Build history of the part. All positions in model axes, mm. A direction names the side the tool comes from. Give positions to 0.01 mm unless a question says otherwise; leave off trailing zeros. Write each loop counter-clockwise with the first axis right and the second up, starting at its lowest first coordinate (ties: lowest second). Pieces come first, ordered by that corner, then holes. Notation, with made-up numbers: M -4.5,67 L 17.5,67 A14 ccw 17.5,71 Z; hole C 63.5,-15.5 d6. An arc over 180 degrees is marked long. One line per item, written item: value. Start each with the question number.
Autodesk Inventor part; units mm, degrees
ref_plane "YZ Plane" through (0, 0, 0) normal (1, 0, 0) x (0, 1, 0)
ref_plane "XZ Plane" through (0, 0, 0) normal (0, 1, 0) x (-1, 0, 0)
ref_plane "XY Plane" through (0, 0, 0) normal (0, 0, 1) x (1, 0, 0)
sketch "スケッチ1" plane through (0, 0, 0) normal (0, 0, 1) x (1, 0, 0)
  line L0 (0, 0) -> (27, 0) construction
  line L1 (27, 0) -> (27, 5) construction
  line L2 (27, 5) -> (0, 5) construction
  line L3 (0, 5) -> (0, 0) construction
  line L4 (0, 2.5) -> (27, 2.5) construction
  line L5 (13.5, 5) -> (13.5, 0) construction
  circle A0 centre (3.7, 2.5) radius 1.55
  line L6 (7.5, 5) -> (7.5, 0) construction
  circle A1 centre (23.3, 2.5) radius 1.55
  line L7 (19.5, 5) -> (19.5, 0) construction
  line L8 (7.49, 5.01) -> (9.59, 5.01) construction
  line L9 (19.51, 5.01) -> (19.51, 2.49)
  line L10 (19.51, 2.49) -> (7.49, 2.49)
  line L11 (7.49, 2.49) -> (7.49, 5.01)
  line L12 (7.49, 5.01) -> (19.51, 2.49) construction
  line L13 (19.51, 5.01) -> (7.49, 2.49) construction
  arc A2 (9.59, 5.01) -> (7.49, 5.01) centre (8.54, 5.01) ccw
  arc A3 (19.51, 5.01) -> (17.41, 5.01) centre (18.46, 5.01) ccw
  line L14 (9.59, 5.01) -> (17.41, 5.01)
  line L15 (9.59, 2.49) -> (7.49, 2.49)
  line L16 (17.41, 5.01) -> (19.51, 5.01) construction
  line L17 (27, 7) -> (0, 7) construction
  line L18 (0, 0) -> (0, 7)
  line L19 (12.1912, 35) -> (37.1912, 35) construction
  line L20 (37.1912, 35) -> (37.1912, 40) construction
  line L21 (37.1912, 40) -> (12.1912, 40) construction
  line L22 (12.1912, 40) -> (12.1912, 35) construction
  line L23 (12.1912, 37.5) -> (37.1912, 37.5) construction
  line L24 (24.6912, 40) -> (24.6912, 35) construction
  circle A4 centre (14.8912, 37.5) radius 1.55
  line L25 (18.6912, 40) -> (18.6912, 35) construction
  line L26 (30.6912, 40) -> (30.6912, 35) construction
  circle A5 centre (34.4912, 37.5) radius 1.55
  line L27 (18.6812, 40.01) -> (20.7812, 40.01) construction
  line L28 (30.7012, 40.01) -> (30.7012, 34.99)
  line L29 (30.7012, 34.99) -> (28.6012, 34.99) construction
  line L30 (18.6812, 34.99) -> (18.6812, 40.01)
  line L31 (18.6812, 40.01) -> (30.7012, 34.99) construction
  line L32 (30.7012, 40.01) -> (18.6812, 34.99) construction
  arc A6 (20.7812, 40.01) -> (18.6812, 40.01) centre (19.7312, 40.01) ccw
  arc A7 (18.6812, 34.99) -> (20.7812, 34.99) centre (19.7312, 34.99) ccw
  arc A8 (30.7012, 40.01) -> (28.6012, 40.01) centre (29.6512, 40.01) ccw
  arc A9 (28.6012, 34.99) -> (30.7012, 34.99) centre (29.6512, 34.99) ccw
  line L33 (20.7812, 40.01) -> (28.6012, 40.01)
  line L34 (20.7812, 34.99) -> (18.6812, 34.99) construction
  line L35 (28.6012, 40.01) -> (30.7012, 40.01) construction
  line L36 (28.6012, 34.99) -> (20.7812, 34.99)
  line L37 (12.1912, 73) -> (12.1912, 68) construction
  circle A10 centre (14.8912, 70.5) radius 1.55
  line L38 (37.1912, 68) -> (37.1912, 73) construction
  line L39 (30.6912, 73) -> (30.6912, 68) construction
  circle A11 centre (34.4912, 70.5) radius 1.55
  line L40 (30.7012, 73.01) -> (30.7012, 67.99)
  line L41 (18.6912, 73) -> (18.6912, 68) construction
  line L42 (12.1912, 68) -> (37.1912, 68) construction
  line L43 (37.1912, 73) -> (12.1912, 73) construction
  line L44 (12.1912, 70.5) -> (37.1912, 70.5) construction
  line L45 (24.6912, 73) -> (24.6912, 68) construction
  line L46 (20.7812, 73.01) -> (28.6012, 73.01)
  line L47 (28.6012, 67.99) -> (20.7812, 67.99)
  line L48 (18.6812, 73.01) -> (30.7012, 67.99) construction
  line L49 (30.7012, 73.01) -> (18.6812, 67.99) construction
  arc A12 (30.7012, 73.01) -> (28.6012, 73.01) centre (29.6512, 73.01) ccw
  line L50 (28.6012, 73.01) -> (30.7012, 73.01) construction
  arc A13 (28.6012, 67.99) -> (30.7012, 67.99) centre (29.6512, 67.99) ccw
  line L51 (30.7012, 67.99) -> (28.6012, 67.99) construction
  line L52 (18.6812, 73.01) -> (20.7812, 73.01) construction
  line L53 (20.7812, 67.99) -> (18.6812, 67.99) construction
  arc A14 (20.7812, 73.01) -> (18.6812, 73.01) centre (19.7312, 73.01) ccw
  arc A15 (18.6812, 67.99) -> (20.7812, 67.99) centre (19.7312, 67.99) ccw
  line L54 (18.6812, 67.99) -> (18.6812, 73.01)
  line L55 (27, 0) -> (27, 6.6473)
  line L56 (37.1912, 35) -> (27.1206, 7.3314)
  line L57 (11.8992, 39.6929) -> (0, 7)
  line L58 (37.1912, 35) -> (37.1912, 73)
  line L59 (6.8054, 101.4338) -> (6.7491, 101.3865)
  arc A16 (4.7394, 86.3065) -> (5.3203, 95.7003) centre (-4.8938, 91.617) ccw
  circle A17 centre (-4.8938, 91.617) radius 14.6063 construction
  line L60 (1.0459, 61.9185) -> (-21.5815, 84.5459) construction
  line L61 (-21.5815, 84.5459) -> (-18.0459, 88.0815) construction
  line L62 (-18.0459, 88.0815) -> (4.5815, 65.4541) construction
  line L63 (4.5815, 65.4541) -> (1.0459, 61.9185) construction
  line L64 (1.0459, 61.9185) -> (-18.0459, 88.0815) construction
  line L65 (-21.5815, 84.5459) -> (4.5815, 65.4541) construction
  line L66 (13.8495, 100.8175) -> (37.1912, 73)
  arc A18 (11.8992, 39.6929) -> (5.2055, 80.7796) centre (-28.1256, 54.2607) ccw
  arc A19 (8.344, 97.7899) -> (6.2953, 101.0057) centre (-4.8938, 91.617) ccw construction
  arc A20 (5.0756, 80.942) -> (7.4988, 83.886) centre (-4.8938, 91.617) ccw construction
  circle A21 centre (8.344, 97.7899) radius 1.55
  circle A22 centre (7.4988, 83.886) radius 1.65
  arc A23 (13.8495, 100.8175) -> (6.8054, 101.4338) centre (10.0193, 97.6035) ccw
  arc A24 (6.7491, 101.3865) -> (5.3203, 95.7003) centre (9.9631, 97.5563) ccw
  arc A25 (4.7394, 86.3065) -> (5.2055, 80.7796) centre (9.1182, 83.8926) ccw
  arc A26 (27.1206, 7.3314) -> (27, 6.6473) centre (29, 6.6473) ccw
  arc A27 (7.49, 3.9749) -> (8.9749, 2.49) centre (8.2325, 3.2325) ccw
  arc A28 (18.0251, 2.49) -> (19.51, 3.9749) centre (18.7675, 3.2325) ccw
  line L67 (0, 0) -> (7.5, -0.5)
  line L68 (7.5, -0.5) -> (19.5, -0.5)
  line L69 (27, 0) -> (19.5, -0.5)
  point P0 (24.6912, 37.5)
  point P1 (24.6912, 70.5)
  point P2 (10.6356, 104.6477)
  point P3 (3.5327, 98.6877)
  point P4 (-8.5, 75)
  point P5 (19.51, 3.9749)
  point P6 (18.0251, 2.49)
  point P7 (5.8711, 81.4297)
  dimension "d0" = 27
  dimension "d1" = 5
  dimension "d2" = 3.1
  dimension "d3" = 12
  dimension "d4" = 19.6
  dimension "d9" = 1.05
  dimension "d10" = 7
  dimension "d11" = 25
  dimension "d12" = 5
  dimension "d13" = 3.1
  dimension "d14" = 12
  dimension "d15" = 19.6
  dimension "d16" = 0.01
  dimension "d17" = 0.01
  dimension "d20" = 1.05
  dimension "d22" = 25
  dimension "d23" = 5
  dimension "d24" = 3.1
  dimension "d25" = 12
  dimension "d26" = 19.6
  dimension "d27" = 0.01
  dimension "d28" = 0.01
  dimension "d29" = 1.05
  dimension "d30" = 70
  dimension "d31" = 66
  dimension "d32" = 33
  dimension "d37" = 5
  dimension "d38" = 75
  dimension "d39" = 135
  dimension "d40" = 8.5
  dimension "d46" = 11.8
  dimension "d47" = 32
  dimension "d48" = 50
  dimension "d49" = 6.8
  dimension "d50" = 11
  dimension "d51" = 29.2126
  dimension "d54" = 15
  dimension "d55" = 15
  dimension "d56" = 3.1
  dimension "d57" = 3.3
  dimension "d60" = 5
  dimension "d61" = 2
  dimension "d62" = 1.05
  dimension "d64" = 2.52
  dimension "d65" = 0.01
  dimension "d66" = 0.01
  dimension "d67" = 0.5
  dimension "d69" = 12
extrude "押し出し1" add sketch "スケッチ1" against normal blind 2
fillet "フィレット1" radius 2 5 edges at (37.1912, 73, -1) (37.1912, 35, -1) (0, 7, -1) (27, 0, -1) (0, 0, -1)
equation "\"d12\" = d1"
equation "\"d13\" = d2"
equation "\"d14\" = d3"
equation "\"d15\" = d4"
equation "\"d16\" = d6"
equation "\"d17\" = d6"
equation "\"d22\" = d11"
equation "\"d23\" = d1"
equation "\"d24\" = d2"
equation "\"d25\" = d3"
equation "\"d26\" = d4"
equation "\"d27\" = d6"
equation "\"d28\" = d6"
equation "\"d32\" = 0.5 * d31"
properties part number "Head_side_frame" material "GFRP"
1) Probe line 1 along Y through (x, z) = (25.5, -0.55); line 2 along X through (y, z) = (70.5, -0.8); line 3 along Y through (x, z) = (26, -0.7). List the from-to ranges inside material, lowest first. Write a range as from..to.
2) Tool access for faces 1 (the face through (13.96, 60.81, -0.99)), 2 (the face through (25, 34.99, -1)): list every direction of +Z, -Z, +X, -X, +Y, -Y with a clear straight run to the whole face (end or side of a thin tool).
3) Band-saw the part on D-D (y = 91). List the corners of the cut face in (x, z), then the cut area to 3 significant figures.
4) Band-saw the part on B-B (z = -0.65). Count the separate pieces of the cut face and the enclosed holes in it, then the cut area to 3 significant figures.
5) Band-saw the part on C-C (x = 34.5). List the corners of the cut face in (y, z).
6) Band-saw the part on A-A (x = 29.5). List the corners of the cut face in (y, z), then the cut area to 3 significant figures.
7) Drop flat-ended pins along their axis: P1, Ø0.5, axis at y = 4.5, z = -1, coming from the +X side; P2, Ø0.6, axis at x = 15.5, z = -0.5, coming from the +Y side; P3, Ø1, axis at x = 24, z = -1, coming from the -Y side; P4, Ø3, axis at x = 34.49, y = 37.5, coming from the -Z side. Give the stop position or say it passes through.
8) Mould opens along Y. For faces 3 (the face through (37.191, 54, -1)), 4 (the face through (19.71, 33.94, -0.99)), 5 (the face through (13, -0.5, -1)) say: released by +Y, released by -Y, zero draft, split by the parting line, or undercut.
Model answer:
1. line 1: y = -0.07..34.99, 40.01..67.99, 73.01..86.93
1. line 2: x = 11.25..13.34, 16.44..18.68, 30.7..32.94, 36.04..37.19
1. line 3: y = 0.14..34.99, 40.01..67.99, 73.01..86.34
2. face 1: +Z, -Z, -X
2. face 2: +Z, -Z
3. outline: M 6.09,-2 L 22.09,-2 L 22.09,0 L 6.09,0 Z
3. area: 32.0 mm²
4. separate pieces: 1
4. enclosed holes: 11
4. area: 2,190 mm²
5. outline: M 27.61,-2 L 35.95,-2 L 35.95,0 L 27.61,0 Z; M 39.05,-2 L 68.95,-2 L 68.95,0 L 39.05,0 Z; M 72.05,-2 L 76.21,-2 L 76.21,0 L 72.05,0 Z
6. outline: M 13.87,-2 L 33.95,-2 L 33.95,0 L 13.87,0 Z; M 41.05,-2 L 66.95,-2 L 66.95,0 L 41.05,0 Z; M 74.05,-2 L 82.17,-2 L 82.17,0 L 74.05,0 Z
6. area: 108 mm²
7. P1: stops at x = 27
7. P2: stops at y = 99.21
7. P3: stops at y = -0.23
7. P4: passes through
8. face 3: zero draft
8. face 4: undercut
8. face 5: released by -Y
